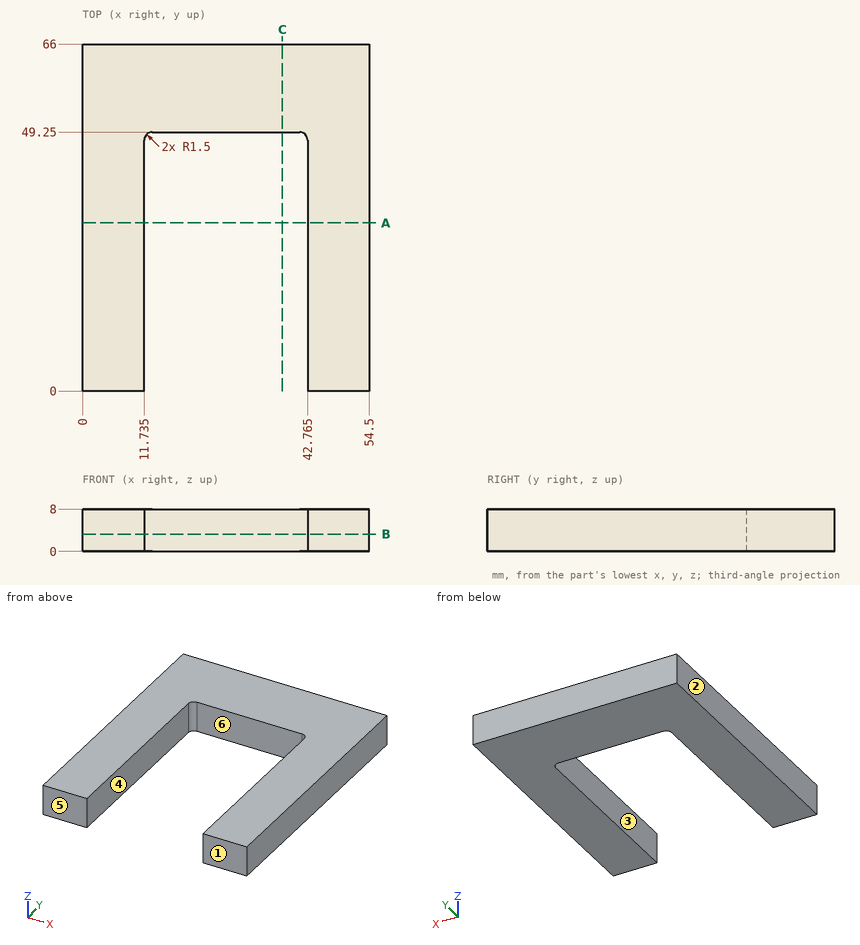
Geometry check sheet. Reference: drawing and pictorial views, mm from the part's lowest x, y, z. A direction names the side the tool comes from. Coordinates: 2 decimals unless noted, no trailing zeros. Order: outer loops, then holes, each group sorted by start corner. A loop starts at its lowest first (then second) coordinate and runs counter-clockwise, first axis right, second up.
1. Set-up check for the marked faces 5 and 6: record each of +Z, -Z, +X, -X, +Y, -Y from which the full face is reachable in a straight line by a thin tool's end or side.
Results found:
face 5: +Z, -Z, +X, -X, -Y
face 6: +Z, -Z, -Y
2. Release check for a two-part mould opening along X. For the marked faces 1, 2, 3 and 4 record: +X half, -X half, draft (parallel to the pull), parting line (faces both ways), or undercut.
Results found:
face 1: draft
face 2: -X half
face 3: undercut
face 4: undercut
3. Sectioned sample at C-C, the plane x = 38. Record the cut outline in (y, z), and give its area (3 significant figures).
Results found:
outline: (49.25, 0) - (66, 0) - (66, 8) - (49.25, 8) - close
area: 134 mm2
4. Go/stop test with a flat-tipped pin: pin 1 Ø4 at (x, z) = (25, 4.5) entering from -Y. Record where the tip stops, or that it passes through.
Results found:
pin 1: stops at y = 49.25
5. Sectioned sample at A-A, the plane y = 32. Record the cut outline in (x, z) (3 decimals).
Results found:
outline: (0, 0) - (11.735, 0) - (11.735, 8) - (0, 8) - close; (42.765, 0) - (54.5, 0) - (54.5, 8) - (42.765, 8) - close
6. Scan lines: line 1 (X direction, y = 32.5, z = 1.75) (3 decimals); line 2 (Y direction, x = 23, z = 2.25); line 3 (X direction, y = 49, z = 2.25). Record each from-to range of solid material in increasing order.
Results found:
line 1: x = 0 to 11.735, 42.765 to 54.5
line 2: y = 49.25 to 66
line 3: x = 0 to 12.41, 42.09 to 54.5
7. Sectioned sample at B-B, the plane z = 3.25. Record the cut outline in (x, y) (3 decimals).
Results found:
outline: (0, 0) - (11.735, 0) - (11.735, 47.75) arc R1.5 cw to (13.235, 49.25) - (41.265, 49.25) arc R1.5 cw to (42.765, 47.75) - (42.765, 0) - (54.5, 0) - (54.5, 66) - (0, 66) - close
